For this review, take the finished solid that the model builds, in its own axes (mm). A direction names the side the tool comes from. Coordinates: 2 decimals unless noted, no trailing zeros. Loops run counter-clockwise (first coordinate to the right, second up) from the corner with the lowest first, then second, coordinate; pieces in that order, holes last. Notation, with made-up numbers: (49, 3.5) - (58, 3.5) arc R23 ccw to (58, 31.5) - close; hole circle Ø10 at (-18, 41). An arc over 180 degrees is marked (long way). Answer as a JSON object with one key per item and string values. Group by question number.
Item 1: We need section A-A (z = -45). Give the boundary of the cut face in (x, y).
Item 2: We need section B-B (z = -18.83). Give the boundary of the cut face in (x, y), then the cut area to 3 significant figures.
Item 3: Tool access review of faces 1 (the flat face through (1.32, 4.15, -26.58)), 2 (the cylindrical face through (1.318, 5.397, -42.802)): name each direction out of +Z, -Z, +X, -X, +Y, -Y from which nothing blocks a thin tool from reaching the whole face with its end or side.
Item 4: Mouldability with a two-part tool opening along Y and no side actions: class faces 3 (the cylindrical face through (1.32, 5.78, -15.06)), 4 (the cylindrical face through (1.282, 0.555, -42.301)), 5 (the cylindrical face through (1.318, 4.803, -16.632)), 6 (the cylindrical face through (1.318, 23.143, -44.862)) as released by +Y, released by -Y, zero draft, split by the parting line, or undercut.
Item 5: We need section C-C (y = 3.5). State how many separate pieces and enclosed holes the cut face has, then the cut area to 3 significant figures.
Item 6: To check wall thickness, follow line 1 (Y direction, x = 1.8, z = -45); line 2 (Y direction, x = 1.3, z = -43.5); line 3 (Z direction, x = 1.7, y = 4). State the ranges of each line that lie inside material, in increasing order.
Item 7: Clearance check with a flat-ended pin moving along its axis: pin 1 (2.5 mm diameter, centred on y = 19.5, z = -44.1, fed in from -X). State where the tip first meets the part, or that it passes through.
Autodesk Inventor part; units mm, degrees
ref_plane "YZ Plane" through (0, 0, 0) normal (1, 0, 0) x (0, 1, 0)
ref_plane "XZ Plane" through (0, 0, 0) normal (0, 1, 0) x (-1, 0, 0)
ref_plane "XY Plane" through (0, 0, 0) normal (0, 0, 1) x (1, 0, 0)
sketch "Boceto1" plane through (0, 0, 0) normal (1, 0, 0) x (0, 1, 0)
  line L0 (0, 0) -> (0, -65)
  line L1 (0, -65) -> (24, -65)
  line L2 (24, -65) -> (24, -45)
  line L3 (24, -45) -> (0, -65)
  line L4 (24, -45) -> (0, 0)
  line L5 (0, -65) -> (0, -60)
  dimension "d0" = 65
  dimension "d6" = 24
  dimension "d7" = 20
  dimension "d8" = 5
extrude "Extrusión1" add sketch "Boceto1" along normal blind 2.6 contours L4 L3 L0
fillet "Empalme1" radius 7 1 edges at (1.3, 0, -65)
fillet "Empalme2" radius 5 1 edges at (1.3, 0, 0)
fillet "Empalme3" radius 3 1 edges at (1.3, 24, -45)
sketch "Boceto2" plane through (2.6, 0, 0) normal (1, 0, 0) x (0, 0, -1)
  line L0 (0, 0) -> (49.1759, 26.2271)
  line L1 (42.8462, 22.8513) -> (17.6471, 9.4118)
  line L2 (0, 0) -> (69.4683, 0)
  arc A0 (50.0547, 0) -> (55.4323, 11.4813) centre (50.0547, 7) ccw
  line L3 (55.4323, 11.4813) -> (45, 24)
  line L4 (55.4323, 11.4813) -> (46.5627, 22.1248)
  line L5 (45, 24) -> (45, 0)
  circle A1 centre (45, 5.3) radius 2.2
  circle A2 centre (44.1, 19.5) radius 2.2
  line L6 (17.6471, 9.4118) -> (20.0129, 0)
  circle A3 centre (18.83, 4.7059) radius 2.2
  dimension "d14" = 4.4
  dimension "d15" = 5.3
  dimension "d18" = 4.4
  dimension "d19" = 0.9
  dimension "d20" = 19.5
  dimension "d21" = 4.4
  dimension "d22" = 26.17
extrude "Extrusión2" cut sketch "Boceto2" against normal blind 10 contours A3 L6 | L6 A3 | A1 L5 | L5 A1 | A2 L5 | L5 A2
sketch "Boceto3" plane through (2.6, 0, 0) normal (1, 0, 0) x (0, 0, -1)
  arc A0 (17.6471, 9.4118) -> (20, 0) centre (20, 5) ccw
  line L0 (55.4323, 11.4813) -> (46.5627, 22.1248)
  line L1 (42.8462, 22.8513) -> (17.6471, 9.4118)
  line L2 (32.6471, 17.4118) -> (36.4118, 10.3529)
  line L3 (20, 0) -> (36.4118, 10.3529)
  line L4 (36.4118, 10.3529) -> (41.9333, 0)
  line L5 (20, 0) -> (50.0547, 0)
  line L6 (20, 0) -> (41.9333, 0)
  point P0 (0, 0)
  dimension "d24" = 90
  dimension "d25" = 8
  dimension "d26" = 17
  dimension "d27" = 11.7333
extrude "Extrusión3" cut sketch "Boceto3" against normal blind 10 contours L3 L4 L5
fillet "Empalme4" radius 4 2 edges at (1.3, 0, -20) (1.3, 0, -41.9333)
fillet "Empalme de cara1" radius 5 1 edges at (1.3, 10.3529, -36.4118)
properties part number "Palanca_barra"
Check sheet entries:
{
 "1": {"outline": "(0, 0) - (2.6, 0) - (2.6, 3.1) - (0, 3.1) - close; (0, 7.5) - (2.6, 7.5) - (2.6, 17.49) - (0, 17.49) - close; (0, 21.51) - (2.6, 21.51) - (2.6, 23.11) - (0, 23.11) - close"},
 "2": {"outline": "(0, 0.31) - (2.6, 0.31) - (2.6, 2.51) - (0, 2.51) - close; (0, 6.91) - (2.6, 6.91) - (2.6, 10.04) - (0, 10.04) - close", "area": "13.9 mm2"},
 "3": {"face 1": "+X, -X, -Y", "face 2": "+X, -X"},
 "4": {"face 3": "split by the parting line", "face 4": "released by -Y", "face 5": "undercut", "face 6": "released by +Y"},
 "5": {"separate pieces": "4", "enclosed holes": "0", "area": "52.4 mm2"},
 "6": {"line 1": "y = 0 to 3.1, 7.5 to 17.49, 21.51 to 23.11", "line 2": "y = 0.09 to 3.69, 6.91 to 17.38, 21.62 to 23.11", "line 3": "z = -56.38 to -46.77, -43.23 to -39.8, -26.34 to -20.91, -16.75 to -15.1"},
 "7": {"pin 1": "passes through"}
}
